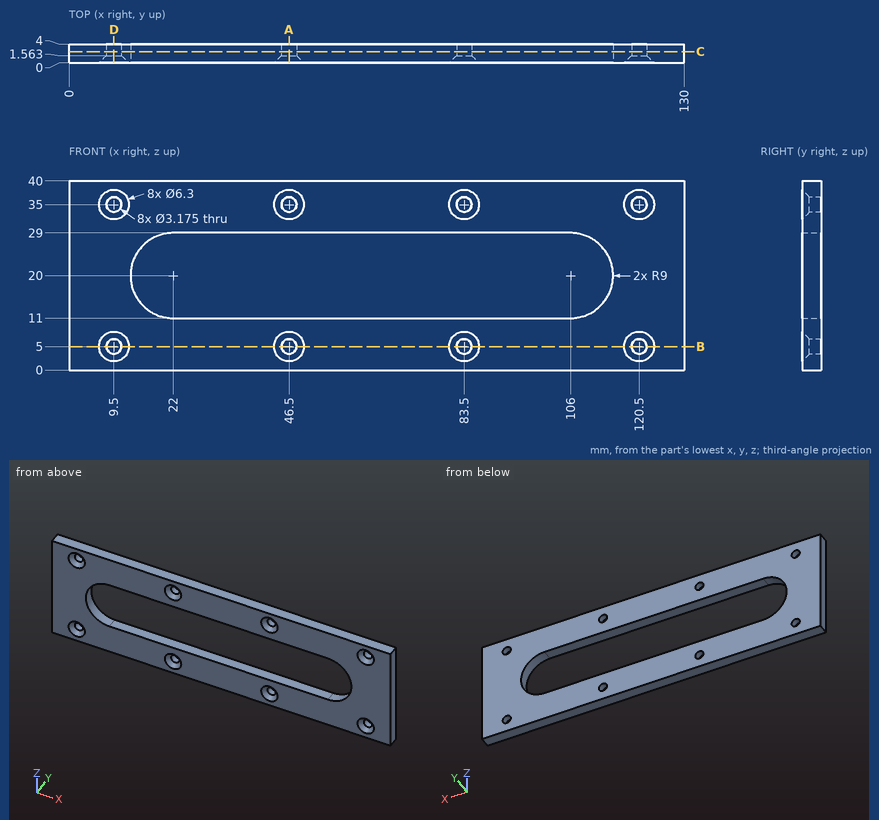
Check sheet for the drawn part. Datum: minimum x, y, z corner. Units: mm. Coordinates: 2 decimals unless noted, no trailing zeros. Order: outer loops, then holes, each group sorted by start corner. A loop starts at its lowest first (then second) coordinate and runs counter-clockwise, first axis right, second up. Notation, with made-up numbers: M 75,-23.75 L 113,-23.75 A17 ccw 113,-19.75 Z; hole C -24.5,-8.5 d1. An arc over 180 degrees is marked long. One line per item, written item: value. Start each with the question number.
Item 1: Sectioned sample at B-B (z = 5). Enter the section's corners in (x, y).
Item 2: Sectioned sample at D-D (x = 9.5). Enter the section's corners in (y, z).
Item 3: Sectioned sample at C-C (y = 2.4). Count the separate pieces of the cut face and the enclosed holes in it, then the cut area to 3 significant figures.
Item 4: Scan lines: probe 1 along X at (y, z) = (3.5, 5); probe 2 along Z at (x, y) = (46.5, 2.3); probe 3 along Z at (x, y) = (61.5, 1.6). Record each from-to range of solid material in increasing order.
Item 5: Sectioned sample at A-A (x = 46.5). Enter the section's corners in (y, z).
Item 6: Gauge pin test, flat ends, axial feed: pin 1 (4 mm diameter, centred on x = 46.5, z = 35, fed in from -Y); pin 2 (5 mm diameter, centred on x = 46.5, z = 5, fed in from -Y). Record the tip position at first contact, or that the pin passes through.
Conclusion:
1. outline: M 0,0 L 6.35,0 L 7.91,1.56 L 7.91,4 L 0,4 Z; M 11.09,1.56 L 12.65,0 L 43.35,0 L 44.91,1.56 L 44.91,4 L 11.09,4 Z; M 48.09,1.56 L 49.65,0 L 80.35,0 L 81.91,1.56 L 81.91,4 L 48.09,4 Z; M 85.09,1.56 L 86.65,0 L 117.35,0 L 118.91,1.56 L 118.91,4 L 85.09,4 Z; M 122.09,1.56 L 123.65,0 L 130,0 L 130,4 L 122.09,4 Z
2. outline: M 0,0 L 4,0 L 4,3.41 L 1.56,3.41 L 0,1.85 Z; M 0,8.15 L 1.56,6.59 L 4,6.59 L 4,33.41 L 1.56,33.41 L 0,31.85 Z; M 0,38.15 L 1.56,36.59 L 4,36.59 L 4,40 L 0,40 Z
3. separate pieces: 1
3. enclosed holes: 9
3. area: 3,370 mm^2
4. probe 1: x = 0 to 7.91, 11.09 to 44.91, 48.09 to 81.91, 85.09 to 118.91, 122.09 to 130
4. probe 2: z = 0 to 3.41, 6.59 to 11, 29 to 33.41, 36.59 to 40
4. probe 3: z = 0 to 11, 29 to 40
5. outline: M 0,0 L 4,0 L 4,3.41 L 1.56,3.41 L 0,1.85 Z; M 0,8.15 L 1.56,6.59 L 4,6.59 L 4,11 L 0,11 Z; M 0,29 L 4,29 L 4,33.41 L 1.56,33.41 L 0,31.85 Z; M 0,38.15 L 1.56,36.59 L 4,36.59 L 4,40 L 0,40 Z
6. pin 1: stops at y = 1.15
6. pin 2: stops at y = 0.65
